Build history of the part. All positions in model axes, mm. A direction names the side the tool comes from. Round coordinates to 2 decimals unless told otherwise and drop trailing zeros. Loops run counter-clockwise (first coordinate to the right, second up) from the corner with the lowest first, then second, coordinate; pieces in that order, holes last. Notation, with made-up numbers: (34, 21.25) - (77, 21.25) arc R35 cw to (77, 53.25) - close; hole circle Ø10 at (22.5, 74.5). An arc over 180 degrees is marked (long way). Put each result on its own line as item: value. Start each with the question number.
from build123d import *

# Parameters (mm, degrees)
SKETCH1_R           = 13
SKETCH1_R_2         = 4
BOSS_EXTRUDE1_DEPTH = 11.5
SKETCH2_R           = 2
BOSS_EXTRUDE2_DEPTH = 3
SKETCH3_R           = 13
SKETCH3_R_2         = 4
BOSS_EXTRUDE3_DEPTH = 11.5


with BuildPart() as part:
    # Sketch1 → Boss-Extrude1 (new body)
    with BuildSketch(Plane.XY):
        Circle(SKETCH1_R)
        Circle(SKETCH1_R_2, mode=Mode.SUBTRACT)
    extrude(amount=BOSS_EXTRUDE1_DEPTH)

    # Sketch2 → Boss-Extrude2 (add)
    with BuildSketch(Plane(origin=(0, 0, 0), x_dir=(-1, 0, 0), z_dir=(0, 0, -1))):
        with Locations((0, 10)):
            Circle(SKETCH2_R)
        with Locations((10, 0)):
            Circle(SKETCH2_R)
        with Locations((0, -10)):
            Circle(SKETCH2_R)
        with Locations((-10, 0)):
            Circle(SKETCH2_R)
    extrude(amount=BOSS_EXTRUDE2_DEPTH)

    # Sketch3 → Boss-Extrude3 (add)
    with BuildSketch(Plane(origin=(0, 0, -3), x_dir=(-1, 0, 0), z_dir=(0, 0, -1))):
        Circle(SKETCH3_R)
        Circle(SKETCH3_R_2, mode=Mode.SUBTRACT)
    extrude(amount=BOSS_EXTRUDE3_DEPTH)


solid = part.part
1) Which spindle directions (+Z, -Z, +X, -X, +Y, -Y) get a long thin tool onto all of the face, cutting with end or side? Do faces 5 (the face through (-10.316, -7.91, 5.67)), 6 (the face through (-3, 3, -3)). Say none if no direction does.
2) Pull direction X, two halves, no side cores. Call faces 1 (the face through (10.316, -7.91, -8.67)), 2 (the face through (0.867, -3.905, -8.67)), 3 (the face through (-3, 3, -14.5)), 4 (the face through (11.6, -1.2, -1.5)): pulls with the +X half, pulls with the -X half, needs draft (parallel to the pull), parting line crosses it, or undercut.
3) Drop flat-ended pins along their axis: pin 1 Ø6.5 at (x, y) = (0, 0) entering from +Z; pin 2 Ø5 at (x, z) = (7.5, -8) entering from -Y; pin 3 Ø8 at (x, z) = (-1.5, -2) entering from +Y; pin 4 Ø5 at (y, z) = (-7.5, 4) entering from -X. Give the stop position or say it passes through.
4) Slice it at B-B, the plane x = 0. Write the cut outline in (y, z).
5) Slice it at C-C, the plane x = -3. Write the cut outline in (y, z).
6) Slice it at A-A, the plane y = 5. Write the cut outline in (x, z).
7) Slice it at D-D, the plane z = -8.5. Write the cut outline in (x, y).
8) Drill centre lines: line 1 (Z direction, x = -6, y = 1); line 2 (X direction, y = 3.5, z = 5); line 3 (Y direction, x = 0, z = 8.25). Where is each one in solid material? Low to high. Write a range as [from, to].
Taken from the geometry:
1. face 5: +Z, -Z
1. face 6: none
2. face 1: parting line crosses it
2. face 2: undercut
2. face 3: needs draft
2. face 4: undercut
3. pin 1: passes through
3. pin 2: stops at y = -12
3. pin 3: stops at y = 13
3. pin 4: stops at x = -12
4. outline: (-13, -14.5) - (-4, -14.5) - (-4, -3) - (-8, -3) - (-8, 0) - (-4, 0) - (-4, 11.5) - (-13, 11.5) - (-13, 0) - (-12, 0) - (-12, -3) - (-13, -3) - close; (4, -14.5) - (13, -14.5) - (13, -3) - (12, -3) - (12, 0) - (13, 0) - (13, 11.5) - (4, 11.5) - (4, 0) - (8, 0) - (8, -3) - (4, -3) - close
5. outline: (-12.65, -14.5) - (-2.65, -14.5) - (-2.65, -3) - (-12.65, -3) - close; (-12.65, 0) - (-2.65, 0) - (-2.65, 11.5) - (-12.65, 11.5) - close; (2.65, -14.5) - (12.65, -14.5) - (12.65, -3) - (2.65, -3) - close; (2.65, 0) - (12.65, 0) - (12.65, 11.5) - (2.65, 11.5) - close
6. outline: (-12, -14.5) - (12, -14.5) - (12, -3) - (-12, -3) - close; (-12, 0) - (12, 0) - (12, 11.5) - (-12, 11.5) - close
7. outline: circle Ø26 at (0, 0); hole circle Ø8 at (0, 0)
8. line 1: z = [-14.5, -3], [0, 11.5]
8. line 2: x = [-12.52, -1.94], [1.94, 12.52]
8. line 3: y = [-13, -4], [4, 13]
